Geometry check sheet. Reference: the model listing, model coordinates, mm. A direction names the side the tool comes from. Coordinates: 2 decimals unless noted, no trailing zeros. Write each loop counter-clockwise with the first axis right and the second up, starting at its lowest first coordinate (ties: lowest second). Pieces come first, ordered by that corner, then holes. Notation, with made-up numbers: (46.5, 40) -> (52.5, 40) arc R23 cw to (52.5, 60) -> close; hole circle Ø1 at (5.5, -21). An arc over 180 degrees is marked (long way). Answer in a Markdown table with one row per item. Add a question column.
1. Scan lines: L1, parallel to Z at x = 4, y = 6.5; L2, parallel to X at y = 20, z = -9.5; L3, parallel to Z at x = -44, y = 25. Record each from-to range of solid material in increasing order. Write a range as from..to.
2. Cross-section at C-C on y = 12.5. Record the cut outline in (x, z), and give its area (3 significant figures).
3. Mould release check, pull along Y, two halves, no side actions. Record for faces 1 (the flat face through (0, 5, -25)), 2 (the flat face through (-1, 18, 12.5)), 3 (the cylindrical face through (56.577, 2.226, -0.245)): pulls with the +Y half, pulls with the -Y half, needs draft (parallel to the pull), parting line crosses it, or undercut.
4. Depth check by flat-ended pin: P1, Ø10, axis at y = 30.5, z = -20.5, coming from the -X side; P2, Ø16, axis at y = 40.5, z = 30.5, coming from the +X side; P3, Ø24, axis at x = 49, y = 16, coming from the +Z side; P4, Ø9, axis at x = -50.5, y = 15.5, coming from the -Z side. Enter the tip coordinate at first touch or a pass-through.
5. Cross-section at D-D on z = -15. Record the cut outline in (x, y), and give its area (3 significant figures).
6. Set-up check for faces 4 (the flat face through (0, 30, -13)), 5 (the flat face through (-20, 27, 27)), 6 (the flat face through (-15, 30, -25)): record each of +Z, -Z, +X, -X, +Y, -Y from which the full face is reachable in a straight line by a thin tool's end or side.
7. Cross-section at A-A on x = 57.5. Record the cut outline in (y, z).
8. Cross-section at B-B on y = 37. Record the cut outline in (x, z), and give its area (3 significant figures).
```python
from build123d import *

# Parameters (mm, degrees)
SKETCH1_W           = 130
SKETCH1_H           = 35
BOSS_EXTRUDE1_DEPTH = 30
SKETCH2_W           = 120
SKETCH2_H           = 25
CUT_EXTRUDE1_DEPTH  = 25
SKETCH3_R           = 2
CUT_EXTRUDE2_DEPTH  = 80.686887253
SKETCH4_R           = 2
CUT_EXTRUDE3_DEPTH  = 80.686887253
SKETCH6_W           = 40
SKETCH6_H           = 55
BOSS_EXTRUDE2_DEPTH = 20
SKETCH7_W           = 30
SKETCH7_H           = 15
CUT_EXTRUDE4_DEPTH  = 50
SKETCH8_W           = 40
SKETCH8_H           = 55
BOSS_EXTRUDE3_DEPTH = 20
SKETCH9_W           = 30
SKETCH9_H           = 15
CUT_EXTRUDE5_DEPTH  = 50


with BuildPart() as part:
    # Sketch1 → Boss-Extrude1 (new body)
    with BuildSketch(Plane(origin=(0, 0, 0), x_dir=(1, 0, 0), z_dir=(0, 1, 0))):
        Rectangle(SKETCH1_W, SKETCH1_H)
    extrude(amount=BOSS_EXTRUDE1_DEPTH)

    # Sketch2 → Cut-Extrude1 (cut)
    with BuildSketch(Plane(origin=(0, 30, 0), x_dir=(1, 0, 0), z_dir=(0, 1, 0))):
        Rectangle(SKETCH2_W, SKETCH2_H)
    extrude(amount=-CUT_EXTRUDE1_DEPTH, mode=Mode.SUBTRACT)

    # Sketch3 → Cut-Extrude2 (cut, through all)
    with BuildSketch(Plane.XY.offset(17.5)):
        with Locations((-57.5, 4)):
            Circle(SKETCH3_R)
    extrude(amount=-CUT_EXTRUDE2_DEPTH, mode=Mode.SUBTRACT)

    # Sketch4 → Cut-Extrude3 (cut, through all)
    with BuildSketch(Plane(origin=(0, 0, -17.5), x_dir=(-1, 0, 0), z_dir=(0, 0, -1))):
        with Locations((-57.5, 4)):
            Circle(SKETCH4_R)
    extrude(amount=-CUT_EXTRUDE3_DEPTH, mode=Mode.SUBTRACT)

    # Sketch6 → Boss-Extrude2 (add)
    with BuildSketch(Plane(origin=(0, 0, -17.5), x_dir=(-1, 0, 0), z_dir=(0, 0, -1))):
        with Locations((0, 27.5)):
            Rectangle(SKETCH6_W, SKETCH6_H)
    extrude(amount=BOSS_EXTRUDE2_DEPTH)

    # Sketch7 → Cut-Extrude4 (cut)
    with BuildSketch(Plane(origin=(0, 55, 0), x_dir=(1, 0, 0), z_dir=(0, 1, 0))):
        with Locations((0, 25)):
            Rectangle(SKETCH7_W, SKETCH7_H)
    extrude(amount=-CUT_EXTRUDE4_DEPTH, mode=Mode.SUBTRACT)

    # Sketch8 → Boss-Extrude3 (add)
    with BuildSketch(Plane.XY.offset(17.5)):
        with Locations((0, 27.5)):
            Rectangle(SKETCH8_W, SKETCH8_H)
    extrude(amount=BOSS_EXTRUDE3_DEPTH)

    # Sketch9 → Cut-Extrude5 (cut)
    with BuildSketch(Plane(origin=(0, 55, 0), x_dir=(1, 0, 0), z_dir=(0, 1, 0))):
        with Locations((0, -25)):
            Rectangle(SKETCH9_W, SKETCH9_H)
    extrude(amount=-CUT_EXTRUDE5_DEPTH, mode=Mode.SUBTRACT)


solid = part.part
```
Results found:
| question | item | result |
|---|---|---|
| 1 | L1 | z = -37.5..-32.5, -17.5..-12.5, 12.5..17.5, 32.5..37.5 |
| 1 | L2 | x = -65..-60, 60..65 |
| 1 | L3 | z = -17.5..-12.5, 12.5..17.5 |
| 2 | outline | (-65, -17.5) -> (-20, -17.5) -> (-20, -37.5) -> (20, -37.5) -> (20, -17.5) -> (65, -17.5) -> (65, 17.5) -> (20, 17.5) -> (20, 37.5) -> (-20, 37.5) -> (-20, 17.5) -> (-65, 17.5) -> close; hole (-60, -12.5) -> (60, -12.5) -> (60, 12.5) -> (-60, 12.5) -> close; hole (-15, -32.5) -> (15, -32.5) -> (15, -17.5) -> (-15, -17.5) -> close; hole (-15, 17.5) -> (15, 17.5) -> (15, 32.5) -> (-15, 32.5) -> close |
| 2 | area | 2,250 mm^2 |
| 3 | face 1 | pulls with the +Y half |
| 3 | face 2 | needs draft |
| 3 | face 3 | undercut |
| 4 | P1 | stops at x = -65 |
| 4 | P2 | stops at x = 20 |
| 4 | P3 | stops at z = 17.5 |
| 4 | P4 | stops at z = -17.5 |
| 5 | outline | (-65, 0) -> (65, 0) -> (65, 30) -> (-65, 30) -> close; hole circle Ø4 at (-57.5, 4); hole circle Ø4 at (57.5, 4) |
| 5 | area | 3,870 mm^2 |
| 6 | face 4 | +X, -X, +Y |
| 6 | face 5 | +Z, -X, +Y, -Y |
| 6 | face 6 | +Y |
| 7 | outline | (0, -17.5) -> (2, -17.5) -> (2, 17.5) -> (0, 17.5) -> close; (6, -17.5) -> (30, -17.5) -> (30, -12.5) -> (6, -12.5) -> close; (6, 12.5) -> (30, 12.5) -> (30, 17.5) -> (6, 17.5) -> close |
| 8 | outline | (-20, -37.5) -> (20, -37.5) -> (20, -17.5) -> (15, -17.5) -> (15, -32.5) -> (-15, -32.5) -> (-15, -17.5) -> (-20, -17.5) -> close; (-20, 17.5) -> (-15, 17.5) -> (-15, 32.5) -> (15, 32.5) -> (15, 17.5) -> (20, 17.5) -> (20, 37.5) -> (-20, 37.5) -> close |
| 8 | area | 700 mm^2 |
